Input: part model. Units: mm. Frame: model coordinates. A direction names the side the tool comes from. Give positions to 0.01 mm unless a question says otherwise; leave off trailing zeros. Loops run counter-clockwise (first coordinate to the right, second up) from the corner with the lowest first, then second, coordinate; pieces in that order, holes last. Notation, with made-up numbers: (65.5, 72.5) -> (120.5, 72.5) arc R8 ccw to (120.5, 82.5) -> close; hole circle Ø11 at (61, 29). An arc over 180 degrees is marked (long way). Answer as a JSON object with one key per item and string values.
```python
from build123d import *

# Parameters (mm, degrees)
F0_W     = 3.8553732447
F0_H     = 10.2907596156
F2_T     = -2.5
F3_DEPTH = 16.3


with BuildPart() as f1:
    # F0 (on Front) → F1 (revolve)
    with BuildSketch(Plane.XZ):
        Rectangle(F0_W, F0_H)
    revolve(axis=Axis((1.9276866224, 0, 0), (0, 0, -1)))

    # F2
    f2_openings = [f1.faces().sort_by_distance(p)[0] for p in [
        (1.927687, 0, 5.14538),
    ]]
    offset(amount=F2_T, openings=f2_openings)

    # F3 (add): a face of the model
    f3_faces = [f1.faces().sort_by_distance(p)[0] for p in [
        (1.9276866224, 0, -2.6453798078),
    ]]
    extrude(f3_faces, amount=F3_DEPTH)


solid = f1.part
```
Q1. Section C-C, the plane z = 3. Return the cut outline in (x, y).
Evaluation:
{"outline": "circle Ø7.71 at (1.93, 0)"}
Q2. Section A-A, the plane y = 0. Return the cut outline in (x, z), then the cut area to 3 significant figures.
Evaluation:
{"outline": "(-1.93, -5.15) -> (5.78, -5.15) -> (5.78, 5.15) -> (3.28, 5.15) -> (3.28, 13.65) -> (0.57, 13.65) -> (0.57, 5.15) -> (-1.93, 5.15) -> close", "area": "102 mm2"}
Q3. Access query for faces 1 (the flat face through (2, 0, -5.145)), 2 (the cylindrical face through (0.676, 0.519, 9.34)). Directions: +Z, -Z, +X, -X, +Y, -Y. A direction counts if a zero-diameter tool reaches every point of the face in a straight line with its end or side. Return the directions, or none.
Evaluation:
{"face 1": "-Z, +X, -X, +Y, -Y", "face 2": "+Z"}
Q4. Section D-D, the plane x = 3.75. Return the cut outline in (y, z).
Evaluation:
{"outline": "(-3.4, -5.15) -> (3.4, -5.15) -> (3.4, 5.15) -> (-3.4, 5.15) -> close"}
Q5. Section B-B, the plane x = 2.5. Return the cut outline in (y, z).
Evaluation:
{"outline": "(-3.81, -5.15) -> (3.81, -5.15) -> (3.81, 5.15) -> (1.23, 5.15) -> (1.23, 13.65) -> (-1.23, 13.65) -> (-1.23, 5.15) -> (-3.81, 5.15) -> close"}
Q6. Ray query, line 1 along Z through (x, y) = (0, 2.75); line 2 along X through (y, z) = (1.5, 3.5); line 3 along Y through (x, z) = (0.75, 9.5). Return the intervals inside material, ascending.
Evaluation:
{"line 1": "z = -5.15 to 5.15", "line 2": "x = -1.62 to 5.48", "line 3": "y = -0.67 to 0.67"}
Q7. Pin query (flat end, axial travel): pin 1 (3 mm diameter, centred on x = 1, z = 9.5, fed in from +Y); pin 2 (1 mm diameter, centred on x = 2.5, y = -2.5, fed in from +Z); pin 3 (4 mm diameter, centred on x = 5, z = 10.5, fed in from +Y). Return the tip coordinate at first contact, or that it passes through.
Evaluation:
{"pin 1": "stops at y = 1.36", "pin 2": "stops at z = 5.15", "pin 3": "stops at y = 0.83"}
